Autodesk Inventor part; units mm, degrees
ref_plane "YZ Plane" through (0, 0, 0) normal (1, 0, 0) x (0, 1, 0)
ref_plane "XZ Plane" through (0, 0, 0) normal (0, 1, 0) x (-1, 0, 0)
ref_plane "XY Plane" through (0, 0, 0) normal (0, 0, 1) x (1, 0, 0)
sketch "Sketch1" plane through (0, 0, 0) normal (0, 0, 1) x (1, 0, 0)
  circle A0 centre (17.0691, -3) radius 1.6
  circle A1 centre (3.0691, -3) radius 1.6
  line L0 (20.1383, 1) -> (0, 1)
  line L1 (0, 1) -> (0, -7)
  line L2 (0, -7) -> (20.1383, -7)
  line L3 (20.1383, 1) -> (20.1383, -7)
  circle A2 centre (17.0691, -82) radius 1.6
  circle A3 centre (3.0691, -82) radius 1.6
  line L4 (20.1383, -86) -> (0, -86)
  line L5 (20.1383, -86) -> (20.1383, -78)
  line L6 (0, -78) -> (20.1383, -78)
  line L7 (0, -86) -> (0, -78)
  circle A4 centre (3.0691, -3) radius 1
  circle A5 centre (17.0691, -3) radius 1
  circle A6 centre (3.0691, -82) radius 1
  circle A7 centre (17.0691, -82) radius 1
  point P0 (0, 0)
  dimension "d0" = 2
  dimension "d1" = 2
  dimension "d2" = 2
  dimension "d3" = 2
extrude "Extrusion1" add sketch "Sketch1" along normal blind 2 contours A0 | A1 | L3 L2 L1 L0 | A2 | A3 | L4 L7 L6 L5
sketch "Sketch2" plane through (0, 0, 2) normal (0, 0, 1) x (1, 0, 0)
  line L0 (20.1383, -7) -> (20.1383, 1)
  line L1 (20.1383, 1) -> (0, 1)
  line L2 (0, 1) -> (0, -7)
  line L3 (0, -7) -> (20.1383, -7)
  circle A0 centre (17.0691, -3) radius 1
  circle A1 centre (3.0691, -3) radius 1
  line L4 (20.1383, -86) -> (20.1383, -78)
  line L5 (20.1383, -78) -> (0, -78)
  line L6 (0, -78) -> (0, -86)
  line L7 (0, -86) -> (20.1383, -86)
  circle A2 centre (17.0691, -82) radius 1
  circle A3 centre (3.0691, -82) radius 1
  circle A4 centre (3.0691, -3) radius 1
  line L8 (3.0691, -3) -> (17.0691, -3)
  line L9 (3.0691, -82) -> (17.0691, -82)
  line L10 (10.0691, -82) -> (10.0691, -3)
  line L11 (6.5691, 1) -> (13.5691, 1)
  line L12 (13.5691, 1) -> (13.5691, -86)
  line L13 (13.5691, -86) -> (6.5691, -86)
  line L14 (6.5691, -86) -> (6.5691, 1)
  line L15 (6.5691, 1) -> (13.5691, -86) construction
  line L16 (13.5691, 1) -> (6.5691, -86) construction
  point P0 (0, 0)
  point P1 (10.0691, -42.5)
  dimension "d6" = 7
  dimension "d7" = 87
extrude "Extrusion2" add sketch "Sketch2" along normal blind 3.5 contours L12 L5 L10 L3 | L3 L10 L8 L12 | L12 L8 L14 L1 | L10 L5 L14 L3 | L3 L14 L8 L10 | L12 L9 L10 L5 | L10 L9 L14 L5 | L12 L7 L14 L9
fillet "Fillet1" radius 2 2 edges at (10.0691, -7, 2) (10.0691, -78, 2)
fillet "Fillet2" radius 2 8 edges at (13.5691, -7, 1.0003) (13.5691, -3, 2) (6.5691, -3, 2) (6.5691, -7, 1.0003) (6.5691, -78, 1.0003) (6.5691, -82, 2) (13.5691, -78, 1.0003) (13.5691, -82, 2)
chamfer "Chamfer1" distance 2 angle 45 8 edges at (20.1383, -86, 1) (20.1383, -78, 1) (0, -86, 1) (0, -78, 1) (20.1383, -7, 1) (20.1383, 1, 1) (0, -7, 1) (0, 1, 1)
chamfer "Chamfer2" distance 3 angle 70 1 edges at (10.0691, -86, 5.5) measured on face at (11.6131, -86, 0.7327)
chamfer "Chamfer3" distance 3 angle 70 1 edges at (10.0691, 1, 5.5) measured on face at (11.6131, 1, 0.7327)
sketch "Sketch3" plane through (0, 0, 5.5) normal (0, 0, 1) x (1, 0, 0)
  line L0 (6.5691, -7.2424) -> (13.5691, -7.2424)
  line L1 (6.5691, -7.2424) -> (6.5691, -77.7576)
  line L2 (13.5691, -77.7576) -> (6.5691, -77.7576)
  line L3 (13.5691, -77.7576) -> (13.5691, -7.2424)
  line L4 (13.5691, -77.7576) -> (6.5691, -77.7576)
  line L5 (10.0691, -77.7576) -> (10.0691, -7.2424)
  circle A0 centre (10.0691, -42.5) radius 1
  line L6 (10.0691, -42.5) -> (10.0691, -27.5)
  circle A1 centre (10.0691, -27.5) radius 1
  line L7 (10.0691, -42.5) -> (10.0691, -57.5)
  circle A2 centre (10.0691, -57.5) radius 1
  point P0 (0, 0)
  dimension "d21" = 2
  dimension "d22" = 15
  dimension "d23" = 2
  dimension "d24" = 15
  dimension "d25" = 2
extrude "Extrusion3" cut sketch "Sketch3" against normal blind 3.5 contours A1 L5 | L5 A1 | A2 L5 | L5 A2 | A0 L5 | L5 A0
properties part number "en_shell_1_wid"
Design review of the part built by this model. Coordinates are the model's own, in mm. A direction names the side the tool comes from. Round coordinates to 2 decimals unless told otherwise and drop trailing zeros. Write each loop counter-clockwise with the first axis right and the second up, starting at its lowest first coordinate (ties: lowest second). Pieces come first, ordered by that corner, then holes.
Item 1: Clearance check with flat-ended pins moving along their axes: pin 1 Ø2.5 at (x, y) = (1.5, -82.5) entering from +Z; pin 2 Ø5.5 at (x, y) = (11.5, -46.5) entering from -Z; pin 3 Ø3 at (y, z) = (-53, 4) entering from +X. State where each tip first meets the part, or that it passes through.
Item 2: For probe 1 along X at (y, z) = (-82, 0.9); probe 2 along X at (y, z) = (-42.5, 4.45); probe 3 along Z at (x, y) = (7.75, -13), list the stretches that pass through material, from the lowest coordinate up.
Item 3: The part is to be moulded in two halves that separate along Y. For faces 6 (the flat face through (18.3, -2.9, 2)), 7 (the flat face through (10.01, -3.18, 4.02)), 8 (the cylindrical face through (2.94, -3.99, 0.99)), say which applies: +Y half, -Y half, draft (parallel to the pull), parting line (faces both ways), or undercut.
Item 4: We need section A-A on y = -27.5. Write out the cut boundary in (x, z), and give its area (3 significant figures).
Item 5: For faces 1 (the flat face through (20.138, -3, 1)), 2 (the flat face through (8, -42, 2)), 3 (the flat face through (10, -82, 0)), 4 (the cylindrical face through (14.14, -7.6, 1.97)), 5 (the flat face through (1.7, -2.9, 2)), list the 3-axis set-ups (+Z, -Z, +X, -X, +Y, -Y) from which the entire face can be reached by the end or side of a thin tool; tool diameter is ignored.
Returned:
1. pin 1: stops at z = 2
1. pin 2: stops at z = 2
1. pin 3: stops at x = 13.57
2. probe 1: x = 0 to 2.07, 4.07 to 16.07, 18.07 to 20.14
2. probe 2: x = 6.57 to 9.07, 11.07 to 13.57
2. probe 3: z = 2 to 5.5
3. face 6: draft
3. face 7: +Y half
3. face 8: undercut
4. outline: (6.57, 2) - (9.07, 2) - (9.07, 5.5) - (6.57, 5.5) - close; (11.07, 2) - (13.57, 2) - (13.57, 5.5) - (11.07, 5.5) - close
4. area: 17.5 mm2
5. face 1: +Z, -Z, +X, +Y, -Y
5. face 2: -Z, +X, -X
5. face 3: -Z, +X, -X, +Y, -Y
5. face 4: +Z, -Z, +X
5. face 5: +Z, -X, +Y, -Y
